from build123d import *

# Parameters (mm, degrees)
BOSS_EXTRUDE1_DEPTH      = 2.54
BOSS_EXTRUDE1_DEPTH_BACK = 12.7
SKETCH1_R                = 18.796
SKETCH2_R                = 18.796
BOSS_EXTRUDE2_DEPTH      = 12.7
BOSS_EXTRUDE3_DEPTH      = 12.7
BOSS_EXTRUDE5_DEPTH      = 12.7
BOSS_EXTRUDE6_DEPTH      = 12.7
SKETCH7_R                = 18.796
BOSS_EXTRUDE7_DEPTH      = 12.7
BOSS_EXTRUDE8_DEPTH      = 25.4
SKETCH11_R               = 12.652854813
BOSS_EXTRUDE10_DEPTH     = 25.4
SKETCH12_R               = 3.250000001
CUT_EXTRUDE2_DEPTH       = 512.464850261
FILLET1_R                = 20.32
BOSS_EXTRUDE11_START     = 114.3
BOSS_EXTRUDE11_DEPTH     = 114.3
SKETCH16_W               = 13.01344698
SKETCH16_H               = 28.816569003
CUT_EXTRUDE4_DEPTH       = 54.61


with BuildPart() as part:
    # Sketch1 → Boss-Extrude1 (new, two sides: drawn at the far end of the back side and taken through both)
    with BuildSketch(Plane.XY.offset(-BOSS_EXTRUDE1_DEPTH_BACK)):
        with Locations((0, -407.299625141)):
            Circle(SKETCH1_R)
    extrude(amount=BOSS_EXTRUDE1_DEPTH + BOSS_EXTRUDE1_DEPTH_BACK)



with BuildPart() as body_2:
    # Sketch2 → Boss-Extrude2 (new body)
    with BuildSketch(Plane(origin=(0, 0, -12.7), x_dir=(-1, 0, 0), z_dir=(0, 0, -1))):
        with BuildLine():
            Line((-26.564149005, -405.379934257), (-31.63093582, -405.013776678))
            ThreePointArc((-31.63093582, -405.013776678), (-3.317825996, -438.839016934), (31.414187958, -411.645887785))
            Line((31.414187958, -411.645887785), (26.382120799, -410.949683715))
            ThreePointArc((26.382120799, -410.949683715), (2.786361575, -380.812356225), (-26.564149005, -405.379934257))
        make_face()
        with Locations(Location((0, -407.299625141, 0), (0, 0, 180))):
            Circle(SKETCH2_R, mode=Mode.SUBTRACT)
    extrude(amount=BOSS_EXTRUDE2_DEPTH)

    # Sketch3 → Boss-Extrude3 (add)
    with BuildSketch(Plane(origin=(0, 0, -25.4), x_dir=(-1, 0, 0), z_dir=(0, 0, -1))):
        with BuildLine():
            Line((14.213346722, -471.208070579), (-197.266538305, -455.67583119))
            Line((-197.266538305, -455.67583119), (-197.266538305, -453.387916788))
            ThreePointArc((-197.266538305, -453.387916788), (-194.645764338, -447.637078669), (-188.586186842, -445.842053367))
            add(Edge.make_bspline(
                [(-31.668722049, -408.98285055), (-77.209858947, -441.706865094), (-129.780268895, -454.105513447), (-188.586186842, -445.842053367)],
                knots=[0, 0, 0, 0, 0.953344593, 0.953344593, 0.953344593, 0.953344593], degree=3))
            ThreePointArc((-31.668722049, -408.98285055), (-2.599324763, -438.906344597), (30.96823039, -414.134090044))
            add(Edge.make_bspline(
                [(30.96823039, -414.134090044), (32.649949124, -424.470701531), (41.040109499, -436.729451805), (38.639174938, -461.09372409), (31.686044055, -471.208070579), (14.213346722, -471.208070579)],
                knots=[0, 0, 0, 0, 0.443747805, 0.572878395, 1, 1, 1, 1], degree=3))
        make_face()
    extrude(amount=-BOSS_EXTRUDE3_DEPTH)

    # Sketch5 → Boss-Extrude5 (add)
    with BuildSketch(Plane.XY.offset(-12.7)):
        with BuildLine():
            Line((31.63093582, -405.013776678), (27.278929363, -405.328279775))
            ThreePointArc((27.278929363, -405.328279775), (2.861336178, -434.499605748), (-27.092003196, -411.047898425))
            Line((-27.092003196, -411.047898425), (-31.414187958, -411.645887785))
            ThreePointArc((-31.414187958, -411.645887785), (3.317825996, -438.839016934), (31.63093582, -405.013776678))
        make_face()
    extrude(amount=BOSS_EXTRUDE5_DEPTH)

    # Sketch6 → Boss-Extrude6 (add)
    with BuildSketch(Plane.XY.offset(-12.7)):
        with BuildLine():
            Line((-14.213346722, -471.208070579), (197.266538305, -455.67583119))
            Line((197.266538305, -455.67583119), (197.266538305, -453.387916788))
            ThreePointArc((197.266538305, -453.387916788), (194.645764338, -447.637078669), (188.586186842, -445.842053367))
            add(Edge.make_bspline(
                [(188.586186842, -445.842053367), (129.780268895, -454.105513447), (77.209858947, -441.706865094), (31.668722049, -408.98285055)],
                knots=[0, 0, 0, 0, 0.953344593, 0.953344593, 0.953344593, 0.953344593], degree=3))
            ThreePointArc((31.668722049, -408.98285055), (2.599324763, -438.906344597), (-30.96823039, -414.134090044))
            add(Edge.make_bspline(
                [(-30.96823039, -414.134090044), (-32.649949124, -424.470701531), (-41.040109499, -436.729451805), (-38.639174938, -461.09372409), (-31.686044055, -471.208070579), (-14.213346722, -471.208070579)],
                knots=[0, 0, 0, 0, 0.443747805, 0.572878395, 1, 1, 1, 1], degree=3))
        make_face()
    extrude(amount=BOSS_EXTRUDE6_DEPTH)


with BuildPart() as part_1:
    add(part.part)

    add(body_2.part)  # Boss-Extrude7 merges body 2
    # Sketch7 → Boss-Extrude7 (add)
    with BuildSketch(Plane(origin=(0, 0, -12.7), x_dir=(-1, 0, 0), z_dir=(0, 0, -1))):
        with Locations(Location((0, -407.299625141, 0), (0, 0, 180))):
            Circle(SKETCH7_R)
    extrude(amount=BOSS_EXTRUDE7_DEPTH)

    # Sketch8 → Boss-Extrude8 (add)
    with BuildSketch(Plane.XY):
        with BuildLine():
            ThreePointArc((-58.391711784, -403.636078411), (-67.121824198, -403.800195984), (-67.358685042, -412.528637671))
            add(Edge.make_bspline(
                [(-37.899374688, -457.862620823), (-44.280461027, -439.825230998), (-54.11365555, -424.711188181), (-67.358685042, -412.528637671)],
                knots=[0, 0, 0, 0, 0.648412371, 0.648412371, 0.648412371, 0.648412371], degree=3))
            add(Edge.make_bspline(
                [(-30.96823039, -414.134090044), (-32.649949124, -424.470701531), (-41.040109499, -436.729451805), (-39.512215319, -452.234259992), (-38.376068735, -456.515151772), (-37.899374688, -457.862620823)],
                knots=[0, 0, 0, 0, 0.443747805, 0.572878395, 0.636374771, 0.636374771, 0.636374771, 0.636374771], degree=3))
            add(Edge.make_bspline(
                [(-30.96823039, -414.134090044), (-41.722283963, -415.45839081), (-50.863444428, -411.959053599), (-58.391711784, -403.636078411)],
                knots=[0, 0, 0, 0, 0.680532916, 0.680532916, 0.680532916, 0.680532916], degree=3))
        make_face()
    extrude(amount=-BOSS_EXTRUDE8_DEPTH)

    # Sketch11 → Boss-Extrude10 (add)
    with BuildSketch(Plane.XY):
        with Locations((-62.670851235, -408.28841522)):
            Circle(SKETCH11_R)
    extrude(amount=-BOSS_EXTRUDE10_DEPTH)

    # Sketch12 → Cut-Extrude2 (cut, through all)
    with BuildSketch(Plane.XY):
        with Locations((-62.670851235, -408.28841522)):
            Circle(SKETCH12_R)
    extrude(amount=-CUT_EXTRUDE2_DEPTH, mode=Mode.SUBTRACT)

    # Fillet1
    # the kernel refuses this fillet: 20.32 mm, written as the material it adds along each edge
    with BuildSketch(Plane(origin=(-59.511042023, -420.540367745, -25.4), x_dir=(-0.9997641834800511, -0.021715833635081266, 0), z_dir=(0, 0, 1))) as fillet1_piece_1:
        with BuildLine():
            CenterArc((10.432056933, 19.781724025), FILLET1_R, 214.575044889, 42.207687895)
            Line((-6.299098106, 8.250425267), (-6.633721207, 8.019799292))
            ThreePointArc((-6.633721207, 8.019799292), (-3.573104641, 3.801857042), (-0.310609577, -0.26207375))
            Line((-0.310609577, -0.26207375), (0.09292103, -0.395634481))
            ThreePointArc((0.09292103, -0.395634481), (2.893002714, -0.07122639), (5.693084398, -0.395634481))
            Line((5.693084398, -0.395634481), (5.786005428, 0))
        make_face()
    extrude(amount=25.4)
    with BuildSketch(Plane(origin=(-50.199792551, -410.425569918, -25.4), x_dir=(0.981910282713407, -0.18934676311381016, 0), z_dir=(0, 0, 1))) as fillet1_piece_2:
        with BuildLine():
            CenterArc((13.766955548, 19.469018818), FILLET1_R, 216.757393509, 69.882984253)
            Line((-2.512952914, 7.308962056), (-2.838551084, 7.065760921))
            ThreePointArc((-2.838551084, 7.065760921), (-1.069058095, 3.718918839), (-0.406312291, -0.008442875))
            Line((-0.406312291, -0.008442875), (-0.135668955, -0.383086015))
            ThreePointArc((-0.135668955, -0.383086015), (9.809532931, -2.061533892), (19.702243107, -0.389380376))
            Line((19.702243107, -0.389380376), (19.58586492, 0))
        make_face()
    extrude(amount=25.4)

    # Sketch15 → Boss-Extrude11 (add)
    with BuildSketch(Plane(origin=(0, 0, -25.4), x_dir=(-1, 0, 0), z_dir=(0, 0, -1)).offset(BOSS_EXTRUDE11_START)):
        with BuildLine():
            Line((-197.266538305, -455.67583119), (14.213346722, -471.208070579))
            Line((14.213346722, -471.208070579), (14.702923537, -464.542216029))
            Line((14.702923537, -464.542216029), (-195.926737542, -449.072421737))
            ThreePointArc((-195.926737542, -449.072421737), (-196.923883913, -451.12857155), (-197.266538305, -453.387916788))
            Line((-197.266538305, -453.387916788), (-197.266538305, -455.67583119))
        make_face()
    extrude(amount=-BOSS_EXTRUDE11_DEPTH)

    # Sketch16 → Cut-Extrude4 (cut)
    with BuildSketch(Plane(origin=(-100.744249605, 0, 0), x_dir=(0, 0, -1), z_dir=(1, 0, 0))):
        with Locations((12.7, -408.663339092)):
            Rectangle(SKETCH16_W, SKETCH16_H)
    extrude(amount=CUT_EXTRUDE4_DEPTH, mode=Mode.SUBTRACT)


solid = part_1.part
Here's how the part is built. I have some questions about the finished solid (model axes, mm). A direction names the side the tool comes from. Round coordinates to 2 decimals unless told otherwise and drop trailing zeros. Order: outer loops, then holes, each group sorted by start corner. A loop starts at its lowest first (then second) coordinate and runs counter-clockwise, first axis right, second up. Notation, with made-up numbers: M -7,70 L -2,70 A26 cw -2,100 Z; hole C 68.5,11 d1. An arc over 180 degrees is marked long. Return JSON: item names as keys, results as strings. Group by question number.
1. If we section it at A-A on z = -71.5: List the corners of the cut face in (x, y) for me, then the cut area to 3 significant figures.
2. On a 3-axis mill with a long thin cutter (end or side, diameter ignored), from which of +Z, -Z, +X, -X, +Y, -Y can I reach the whole of each face in a straight line? I mean faces 4 (the face through (3.45, -434.43, -6.44)), 5 (the face through (-53, -423.072, -13)), 6 (the face through (-14.455, -467.922, -83.35)), 7 (the face through (89.137, -456.916, -83.35)). Say none if no direction works.
3. If we section it at B-B on x = 0: List the corners of the cut face in (y, z) for me.
4. Please list where these lines run through material, in increasing order: probe 1 along Z at (x, y) = (-36.5, -421); probe 2 along X at (y, z) = (-412, -9); probe 3 along Y at (x, z) = (185, -62.5).
5. I'm going to push flat-ended pins straight in: pin 1 Ø8 at (x, y) = (-56.5, -412) entering from +Z; pin 2 Ø10.5 at (y, z) = (-413.5, -13) entering from -X; pin 3 Ø2 at (x, y) = (-9, -427) entering from +Z. Where does each tip first touch, or does it pass through?
6. If we mould it in two halves opening along X, with no side actions, what happens to faces 1 (the face through (-56.98, -424.55, -12.88)), 2 (the face through (7, -425, -12.7)), 3 (the face through (-61, -413, -19.207))? For each: pulls with the +X half, pulls with the -X half, needs draft (parallel to the pull), parting line crosses it, or undercut.
Reply:
{
 "1": {"outline": "M -14.7,-464.54 L -14.21,-471.21 L 197.27,-455.68 L 197.27,-453.39 A7.62 ccw 195.93,-449.07 Z", "area": "1,420 mm^2"},
 "2": {"face 4": "+Z", "face 5": "-X, +Y", "face 6": "-Z, -X, -Y", "face 7": "-Z, -X, +Y"},
 "3": {"outline": "M -470.16,-139.7 L -463.46,-139.7 L -463.46,-25.4 L -380.67,-25.4 L -380.67,-12.7 L -388.5,-12.7 L -388.5,2.54 L -426.1,2.54 L -426.1,-12.7 L -434.65,-12.7 L -434.65,0 L -470.16,0 Z"},
 "4": {"probe 1": "-25.4 to 0", "probe 2": "-46.13 to -42.26, -31.36 to -26.94, -18.2 to 18.2, 26.94 to 35.97", "probe 3": "-456.58 to -449.87"},
 "5": {"pin 1": "z = 0", "pin 2": "x = -46.13", "pin 3": "z = -12.7"},
 "6": {"face 1": "pulls with the -X half", "face 2": "undercut", "face 3": "needs draft"}
}
